Here's the drawing with two shaded views (mm, measured from the low corner). I have some questions. A direction names the side the tool comes from. Round coordinates to 2 decimals unless told otherwise and drop trailing zeros. Loops run counter-clockwise (first coordinate to the right, second up) from the corner with the lowest first, then second, coordinate; pieces in that order, holes last.
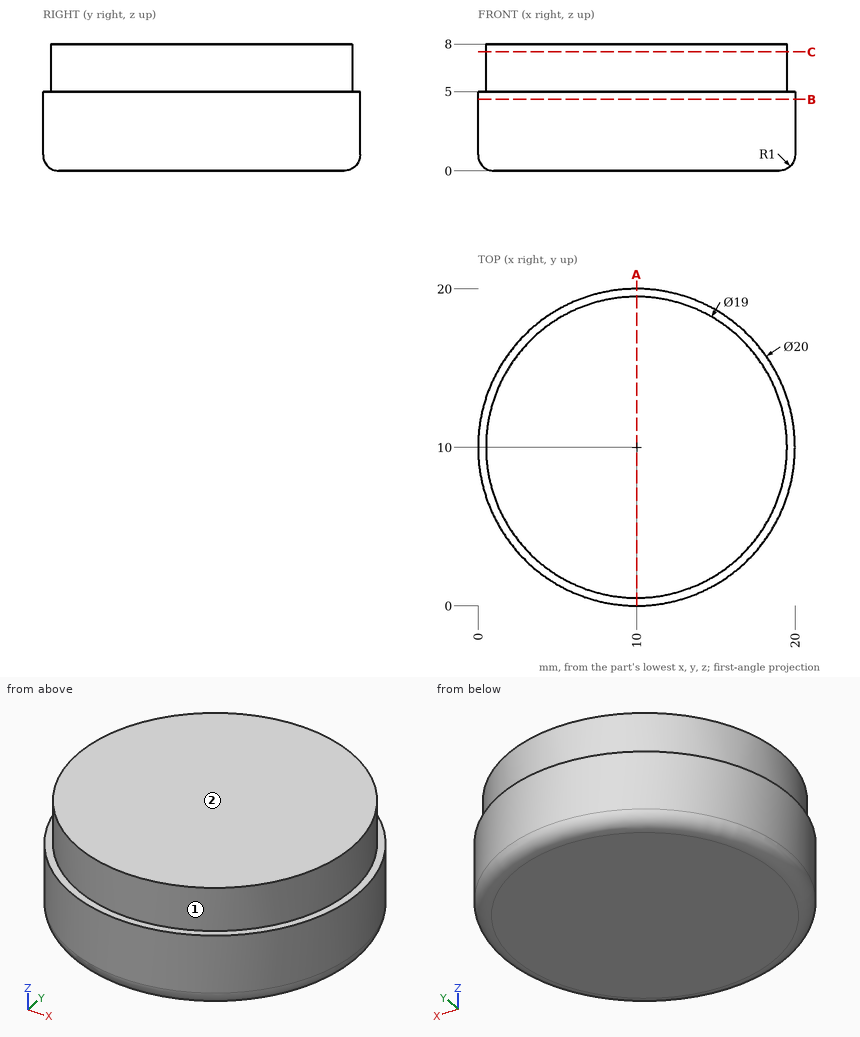
(1) If we section it at B-B, the plane z = 4.5: List the corners of the cut face in (x, y) for me.
Worked answers:
outline: circle Ø20 at (10, 10)
(2) If I drill on line 1 (Y direction, x = 10, z = 2.75); line 2 (X direction, y = 9.75, z = 5.5); line 3 (Y direction, x = 1.5, z = 0.5), over which ranges is the centre line in solid material (lowest first)?
Worked answers:
line 1: y = 0 to 20
line 2: x = 0.5 to 19.5
line 3: y = 4.99 to 15.01
(3) Will this pin go through, and if not, where does the flat tip stop? P1, Ø1, axis at y = 9.5, z = 7, coming from the +X side.
Worked answers:
P1: stops at x = 19.5
(4) If we section it at A-A, the plane x = 10: List the corners of the cut face in (y, z) for me, then the cut area to 3 significant figures.
Worked answers:
outline: (0, 1) arc R1 ccw to (1, 0) - (19, 0) arc R1 ccw to (20, 1) - (20, 5) - (19.5, 5) - (19.5, 8) - (0.5, 8) - (0.5, 5) - (0, 5) - close
area: 157 mm2
(5) If we section it at C-C, the plane z = 7.5: List the corners of the cut face in (x, y) for me, then the cut area to 3 significant figures.
Worked answers:
outline: circle Ø19 at (10, 10)
area: 284 mm2
(6) For the marked faces 1 and 2, which set-ups out of +Z, -Z, +X, -X, +Y, -Y let a thin tool reach every point of the face, with its end or its side?
Worked answers:
face 1: +Z
face 2: +Z, +X, -X, +Y, -Y
